Check sheet for the modelled part. Datum: model origin and axes. Units: mm. Give positions to 0.01 mm unless a question says otherwise; leave off trailing zeros. Order: outer loops, then holes, each group sorted by start corner. A loop starts at its lowest first (then second) coordinate and runs counter-clockwise, first axis right, second up. Notation, with made-up numbers: (79.5, -36) -> (109.5, -36) arc R22 cw to (109.5, -17) -> close; hole circle Ø7 at (0, 79). An arc over 180 degrees is marked (long way). Answer in a Markdown table with one row per item. Add a question column.
(1) Go/stop test with flat-tipped pins: pin 1 (3 mm diameter, centred on x = 34, y = 4.5, fed in from +Z); pin 2 (1 mm diameter, centred on x = 32.5, z = -10, fed in from -Y); pin 3 (6 mm diameter, centred on x = 44.5, y = 17, fed in from +Z). Record where each tip stops, or that it passes through.
(2) Cross-section at A-A (y = 1). Record the cut outline in (x, z), then the cut area to 3 significant figures.
(3) Cross-section at B-B (x = 25.5). Record the cut outline in (y, z), then the cut area to 3 significant figures.
(4) Thickness scan on L1, parallel to Z at x = 47, y = 1.5; L2, parallel to Y at x = 49, z = -14; L3, parallel to X at y = -17, z = -11. Record the ranges inside material, lowest first. Write a range as [from, to].
(5) Cross-section at C-C (z = -15). Record the cut outline in (x, y).
Autodesk Inventor part; units mm, degrees
ref_plane "工作平面1" through (10, 22, 0) normal (-0.3643, -0.6585, -0.6585) x (0.875, 0, -0.4841)
ref_plane "YZ Plane" through (0, 0, 0) normal (1, 0, 0) x (0, 1, 0)
ref_plane "XZ Plane" through (0, 0, 0) normal (0, 1, 0) x (-1, 0, 0)
sketch "草圖1" plane through (0, 0, 0) normal (0, 1, 0) x (-1, 0, 0)
  line L0 (0, 0) -> (-57, 0)
  line L1 (-57, 0) -> (-57, -36)
  line L2 (-57, -36) -> (0, -36)
  line L3 (0, -36) -> (0, 0)
  dimension "d0" = 57
  dimension "d1" = 36
extrude "擠出1" add sketch "草圖1" along normal mid plane 44
sketch "草圖2" plane through (0, 22, 0) normal (0, 1, 0) x (1, 0, 0)
  line L0 (0, 0) -> (57, 0)
  line L1 (10, 0) -> (57, 6)
  line L2 (57, 0) -> (57, 36)
  dimension "d4" = 10
  dimension "d5" = 30
extrude "擠出2" cut sketch "草圖2" against normal blind 60
sketch "草圖3" plane through (57, -22, -36) normal (1, 0, 0) x (0, 0, -1)
  line L0 (-30, 24) -> (-10, 44)
  line L1 (0, 44) -> (-36, 44)
  line L2 (-30, 44) -> (-30, 0)
  point P0 (-36, 22)
  point P1 (-30, 2)
  dimension "d8" = 20
  dimension "d9" = 20
ref_plane "工作平面1" through (10, 22, 0) normal (-0.3643, -0.6585, -0.6585) x (0.875, 0, -0.4841)
sketch "草圖4" plane through (10, 22, 0) normal (-0.3643, -0.6585, -0.6585) x (0.875, 0, -0.4841)
  line L0 (-15.1543, -12.3218) -> (93.717, -12.3218)
  line L1 (93.717, -12.3218) -> (93.717, 28.8166)
  line L2 (93.717, 28.8166) -> (-15.1543, 28.8166)
  line L3 (-15.1543, 28.8166) -> (-15.1543, -12.3218)
  point P0 (-8.7503, 13.3688)
extrude "擠出3" cut sketch "草圖4" against normal blind 40
mirror "鏡射1" about plane through (0, 0, 0) normal (0, 1, 0) of "擠出3"
properties part number "47"
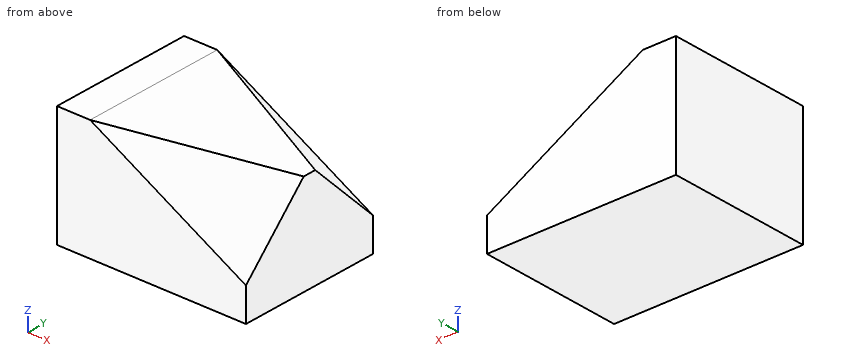
Answer below:
| question | item | result |
|---|---|---|
| 1 | pin 1 | stops at z = -2.87 |
| 1 | pin 2 | stops at y = -20.12 |
| 1 | pin 3 | stops at z = -10.66 |
| 2 | outline | (0, -36) -> (57, -36) -> (57, -6) -> (10, 0) -> (0, 0) -> close |
| 2 | area | 1,910 mm² |
| 3 | outline | (-22, -36) -> (22, -36) -> (22, -8.58) -> (15.4, -1.98) -> (-15.4, -1.98) -> (-22, -8.58) -> close |
| 3 | area | 1,450 mm² |
| 4 | L1 | z = [-36, -4.72] |
| 4 | L2 | y = [-14.42, 14.42] |
| 4 | L3 | x = [0, 38.92] |
| 5 | outline | (0, -22) -> (37.11, -22) -> (57, -11) -> (57, 11) -> (37.11, 22) -> (0, 22) -> close |
